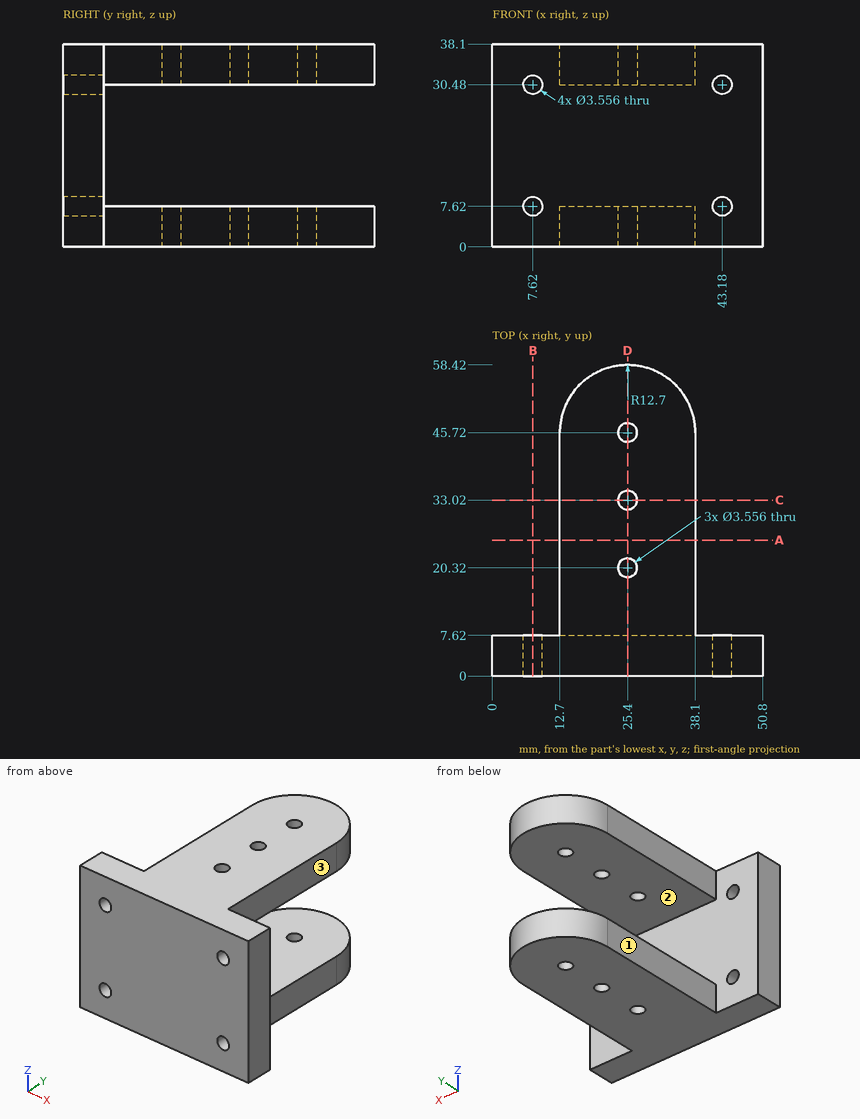
Geometry: see drawing. Coordinates: mm, zero at the bounding-box minimum. A direction names the side the tool comes from. Give positions to 0.01 mm unless a question says otherwise; leave off trailing zeros. Order: outer loops, then holes, each group sorted by start corner. A loop starts at its lowest first (then second) coordinate and runs counter-clockwise, first axis right, second up.
1. Cut plane C-C (y = 33.02). Return loops of the section in (x, z), and give its area (3 significant figures).
Computed:
outline: (12.7, 0) - (23.62, 0) - (23.62, 7.62) - (12.7, 7.62) - close; (12.7, 30.48) - (23.62, 30.48) - (23.62, 38.1) - (12.7, 38.1) - close; (27.18, 0) - (38.1, 0) - (38.1, 7.62) - (27.18, 7.62) - close; (27.18, 30.48) - (38.1, 30.48) - (38.1, 38.1) - (27.18, 38.1) - close
area: 333 mm2
2. Cut plane A-A (y = 25.5). Return loops of the section in (x, z).
Computed:
outline: (12.7, 0) - (38.1, 0) - (38.1, 7.62) - (12.7, 7.62) - close; (12.7, 30.48) - (38.1, 30.48) - (38.1, 38.1) - (12.7, 38.1) - close
3. Line query: probe 1 along Y at (x, z) = (25.4, 2.5); probe 2 along X at (y, z) = (33.02, 4); probe 3 along Z at (x, y) = (37, 22.5). Output: solid intervals per line, ascending.
Computed:
probe 1: y = 0 to 18.54, 22.1 to 31.24, 34.8 to 43.94, 47.5 to 58.42
probe 2: x = 12.7 to 23.62, 27.18 to 38.1
probe 3: z = 0 to 7.62, 30.48 to 38.1
4. Set-up query: the marked faces 1, 2 and 3. Return all of +Z, -Z, +X, -X, +Y, -Y with unobstructed straight access to the full face (end or side cutting, diameter ignored); none if empty.
Computed:
face 1: +Z, -Z, -X, +Y
face 2: +X, -X, +Y
face 3: +Z, -Z, +X, +Y
5. Pin query (flat end, axial travel): pin 1 Ø3 at (x, z) = (43.18, 30.48) entering from -Y; pin 2 Ø6 at (y, z) = (25.5, 35.5) entering from +X; pin 3 Ø4 at (x, z) = (43.18, 7.62) entering from +Y; pin 4 Ø6 at (y, z) = (21, 33.5) entering from -X. Return the tip coordinate at first contact, or that it passes through.
Computed:
pin 1: passes through
pin 2: stops at x = 38.1
pin 3: stops at y = 7.62
pin 4: stops at x = 12.7
6. Cut plane B-B (x = 7.62). Return loops of the section in (y, z), and give its area (3 significant figures).
Computed:
outline: (0, 0) - (7.62, 0) - (7.62, 5.84) - (0, 5.84) - close; (0, 9.4) - (7.62, 9.4) - (7.62, 28.7) - (0, 28.7) - close; (0, 32.26) - (7.62, 32.26) - (7.62, 38.1) - (0, 38.1) - close
area: 236 mm2
7. Cut plane D-D (x = 25.4). State how many separate pieces and enclosed holes the cut face has, and give its area (3 significant figures).
Computed:
separate pieces: 7
enclosed holes: 0
area: 902 mm2
